from build123d import *

# Parameters (mm, degrees)
CUT_EXTRUDE1_REACH = 4.5
SKETCH2_R          = 37.5


with BuildPart() as part:
    # Sketch1 → Revolve1 (revolve)
    with BuildSketch(Plane.XY):
        Polygon((0, 0), (37.5, 0), (37.5, 19.5), (45, 19.5), (45, 17), (40, 17), (40, 0), (45, 0), (45, -2.5), (0, -2.5), align=None)
    revolve(axis=Axis((0, -2.5, 0), (0, 1, 0)))

    # Sketch2 → Cut-Extrude1 (cut, up to next)
    with BuildSketch(Plane(origin=(0, 0, 0), x_dir=(1, 0, 0), z_dir=(0, 1, 0)), mode=Mode.PRIVATE) as cut_extrude1_sk1:
        Circle(SKETCH2_R)
    cut_extrude1_tool1 = extrude(cut_extrude1_sk1.sketch, amount=-CUT_EXTRUDE1_REACH, mode=Mode.PRIVATE) & part.part
    add(cut_extrude1_tool1.solids().sort_by_distance((0, 0, 0))[0], mode=Mode.SUBTRACT)


solid = part.part
Read the model definition and answer for the solid it produces. Units are mm, in the model's axes. A direction names the side the tool comes from. Give positions to 0.01 mm unless a question says otherwise; leave off trailing zeros. Write each loop counter-clockwise with the first axis right and the second up, starting at its lowest first coordinate (ties: lowest second). Pieces come first, ordered by that corner, then holes. Notation, with made-up numbers: M 51.5,85 L 59.5,85 A31 cw 59.5,124 Z; hole C 70,7.25 d5. An arc over 180 degrees is marked long. One line per item, written item: value. Start each with the question number.
(1) Determine the mould class of faces 3 (the flat face through (30.2, 0, 26.5)), 4 (the cylindrical face through (20.765, -1.268, 39.923)), 5 (the flat face through (17, 19.5, -34)), 6 (the flat face through (-17, -2.5, -34)) for opening direction Y: pulls with the +Y half, pulls with the -Y half, needs draft (parallel to the pull), parting line crosses it, or undercut.
(2) Find section A-A (z = 0). Determine the outline of the cut face in (x, y).
(3) Find the intervals of material crossed by line 1 (Z direction, x = 0, y = 4.75); line 2 (Y direction, x = 17.5, z = -37), in increasing order.
(4) Find section B-B (x = 0). Determine the outline of the cut face in (y, z).
(5) Flat-ended cylindrical pins translate along their axes: pin 1 Ø8 at (y, z) = (15.5, -3) entering from -X; pin 2 Ø10 at (x, y) = (21.5, 16.5) entering from +Z; pin 3 Ø4 at (x, y) = (20, 17) entering from +Z; pin 4 Ø8 at (x, y) = (-23.5, 7.5) entering from -Z. Find the tip coordinate at first contact, or state that the pin passes through.
(6) Find section C-C (y = 11.5). Determine the outline of the cut face in (x, z), plus the area to 3 significant figures.
(7) A tool of negligible diameter and unlimited length cuts with its end or side. For faces 1 (the cylindrical face through (-4.88, 8.65, -37.18)), 2 (the flat face through (-30.2, 17, 26.5)), from which of +Z, -Z, +X, -X, +Y, -Y can it reach the whole face along a straight path? Write none if from no direction.
Results below:
1. face 3: undercut
1. face 4: needs draft
1. face 5: pulls with the +Y half
1. face 6: pulls with the -Y half
2. outline: M -45,-2.5 L -37.5,-2.5 L -37.5,19.5 L -45,19.5 L -45,17 L -40,17 L -40,0 L -45,0 Z; M 37.5,-2.5 L 45,-2.5 L 45,0 L 40,0 L 40,17 L 45,17 L 45,19.5 L 37.5,19.5 Z
3. line 1: z = -40 to -37.5, 37.5 to 40
3. line 2: y = -2.5 to 0, 17 to 19.5
4. outline: M -2.5,-45 L 0,-45 L 0,-40 L 17,-40 L 17,-45 L 19.5,-45 L 19.5,-37.5 L -2.5,-37.5 Z; M -2.5,37.5 L 19.5,37.5 L 19.5,45 L 17,45 L 17,40 L 0,40 L 0,45 L -2.5,45 Z
5. pin 1: stops at x = -45
5. pin 2: stops at z = 41.86
5. pin 3: stops at z = 41.24
5. pin 4: stops at z = -34.92
6. outline: C 0,0 d80; hole C 0,0 d75
6. area: 609 mm^2
7. face 1: +Y, -Y
7. face 2: none
